Input: dimensioned drawing with shaded views. Units: mm. Origin: part minimum x, y, z. A direction names the side the tool comes from. Round coordinates to 2 decimals unless told otherwise and drop trailing zeros. Loops run counter-clockwise (first coordinate to the right, second up) from the corner with the lowest first, then second, coordinate; pieces in that order, holes last.
1) Section A-A, the plane x = 43.5. Return loops of the section in (y, z).
2) Section D-D, the plane x = 37.5. Return loops of the section in (y, z).
3) Access query for the marked faces 1 and 2. Directions: +Z, -Z, +X, -X, +Y, -Y. A direction counts if a zero-diameter tool reaches every point of the face in a straight line with its end or side. Return the directions, or none.
4) First-contact query: pin 1 (8 mm diameter, centred on x = 15.5, y = 21, fed in from +Z); pin 2 (22 mm diameter, centred on x = 40.5, y = 12, fed in from +Z); pin 3 (12 mm diameter, centred on x = 36, y = 27, fed in from +Z); pin 4 (2 mm diameter, centred on x = 42.5, y = 7.5, fed in from +Z). Flat tips, straight axial feed; report the tip coordinate or a pass-through.
5) Section C-C, the plane y = 22. Return loops of the section in (x, z), and give its area (3 significant figures).
6) Section B-B, the plane z = 15.5. Return loops of the section in (x, y).
7) Ray query, line 1 along Y through (x, z) = (46, 19.5); line 2 along X through (y, z) = (11.5, 33); line 3 along Z through (x, y) = (17, 9). Return the intervals inside material, ascending.
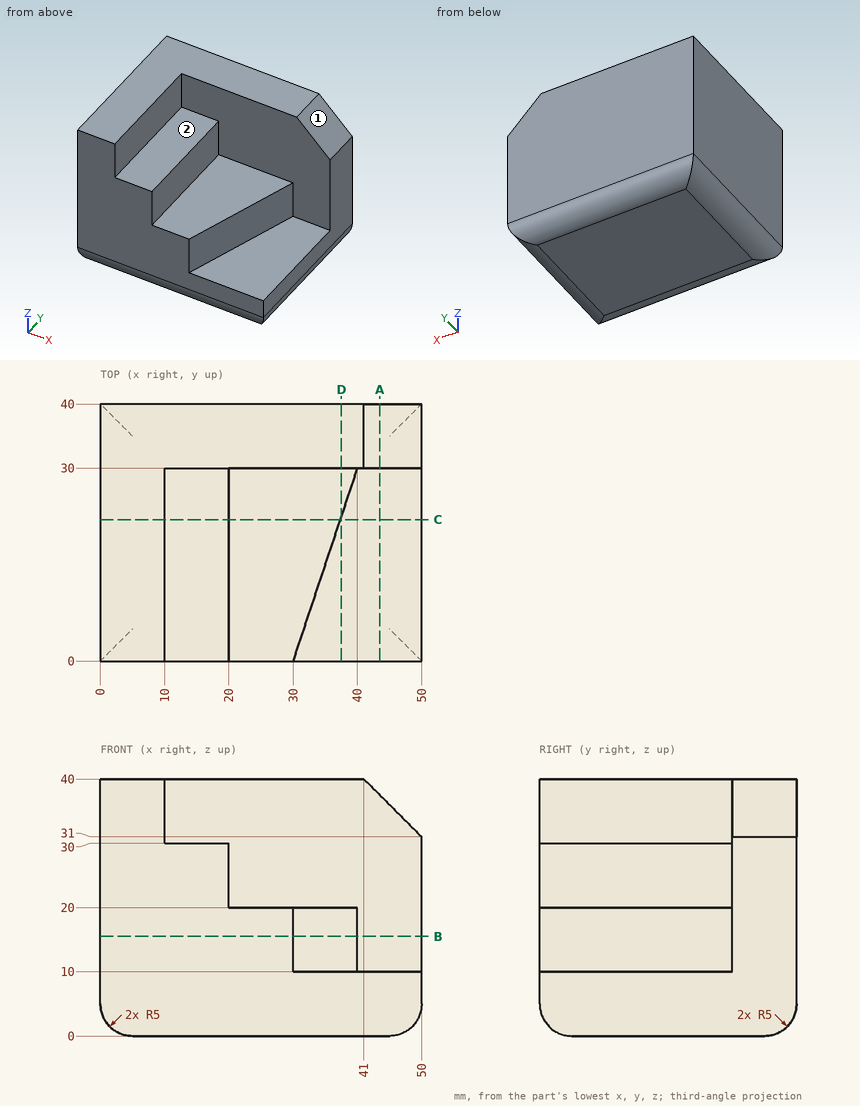
Final values:
1. outline: (0, 5) arc R5 ccw to (5, 0) - (35, 0) arc R5 ccw to (40, 5) - (40, 37.5) - (30, 37.5) - (30, 10) - (0, 10) - close
2. outline: (0, 5) arc R5 ccw to (5, 0) - (35, 0) arc R5 ccw to (40, 5) - (40, 40) - (30, 40) - (30, 20) - (22.5, 20) - (22.5, 10) - (0, 10) - close
3. face 1: +Z, +X, +Y, -Y
3. face 2: +Z, +X, -Y
4. pin 1: stops at z = 30
4. pin 2: stops at z = 20
4. pin 3: stops at z = 40
4. pin 4: stops at z = 10
5. outline: (0, 5) arc R5 ccw to (5, 0) - (45, 0) arc R5 ccw to (50, 5) - (50, 10) - (37.33, 10) - (37.33, 20) - (20, 20) - (20, 30) - (10, 30) - (10, 40) - (0, 40) - close
5. area: 1,160 mm2
6. outline: (0, 0) - (30, 0) - (40, 30) - (50, 30) - (50, 40) - (0, 40) - close
7. line 1: y = 30 to 40
7. line 2: x = 0 to 10
7. line 3: z = 0 to 30
